Work out the finished part from the listing and answer in its coordinate system (mm). A direction names the side the tool comes from. Round coordinates to 2 decimals unless told otherwise and drop trailing zeros.
```python
from build123d import *

# Parameters (mm, degrees)
SKETCH2_W               = 316.892468242
SKETCH2_H               = 286.660554426
CUT_EXTRUDE1_DEPTH      = 1.27
CUT_EXTRUDE1_DEPTH_BACK = 77.2
SKETCH3_R               = 3.175
CUT_EXTRUDE2_DEPTH      = 19.05
CIRPATTERN1_COUNT       = 8


with BuildPart() as part:
    # Sketch1 → Revolve1 (revolve)
    with BuildSketch(Plane(origin=(0, 0, 0), x_dir=(0, 0, -1), z_dir=(1, 0, 0))):
        with BuildLine():
            ThreePointArc((-50.167050753, 76.2), (-43.047460251, 74.691369941), (-37.013141195, 70.623013134))
            Line((-37.013141195, 70.623013134), (-2.24506403, 35.85493597))
            ThreePointArc((-2.24506403, 35.85493597), (0, 34.925), (2.24506403, 35.85493597))
            ThreePointArc((2.24506403, 35.85493597), (21.675043526, 50.270960023), (44.45, 58.434734291))
            Line((44.45, 58.434734291), (44.45, 76.2))
            Line((44.45, 76.2), (30.1625, 76.2))
            Line((30.1625, 76.2), (30.1625, 73.025))
            Line((30.1625, 73.025), (25.4, 73.025))
            Line((25.4, 73.025), (25.4, 76.2))
            Line((25.4, 76.2), (-25.4, 76.2))
            Line((-25.4, 76.2), (-25.4, 73.025))
            Line((-25.4, 73.025), (-30.1625, 73.025))
            Line((-30.1625, 73.025), (-30.1625, 76.2))
            Line((-30.1625, 76.2), (-50.167050753, 76.2))
        make_face()
    revolve(axis=Axis((0, 0, 0), (0, 0, 1)))

    # Sketch2 → Cut-Extrude1 (cut, two sides)
    with BuildSketch(Plane(origin=(0, 0, 0), x_dir=(1, 0, 0), z_dir=(0, 1, 0))) as cut_extrude1_sk:
        Rectangle(SKETCH2_W, SKETCH2_H)
    extrude(amount=CUT_EXTRUDE1_DEPTH, mode=Mode.SUBTRACT)
    extrude(cut_extrude1_sk.sketch, amount=-CUT_EXTRUDE1_DEPTH_BACK, mode=Mode.SUBTRACT)

    # Sketch3 → Cut-Extrude2 (cut)
    with BuildSketch(Plane(origin=(29.160477546, 70.399620377, 0), x_dir=(0, 0, -1), z_dir=(0.382683432, 0.923879533, 0))):
        Circle(SKETCH3_R)
    cut_extrude2 = extrude(amount=-CUT_EXTRUDE2_DEPTH, mode=Mode.SUBTRACT)

    # CirPattern1: Cut-Extrude2 ×8 about axis
    cirpattern1_axis = Axis((0, 0, 0), (0, 0, 1))
    for i in range(1, CIRPATTERN1_COUNT):
        add(cut_extrude2.rotate(cirpattern1_axis, i * 360 / CIRPATTERN1_COUNT), mode=Mode.SUBTRACT)


solid = part.part
```
1. Given pin 1 (3 mm diameter, centred on y = 59, z = -35, fed in from -X); pin 2 (10 mm diameter, centred on x = -29, y = 32.5, fed in from -Z); pin 3 (4 mm diameter, centred on x = 31.5, y = 48.5, fed in from +Z), each flat-ended and moving along its own axis, determine where each tip first touches the part or whether it passes through.
Answer key:
pin 1: stops at x = -50
pin 2: stops at z = -18.63
pin 3: stops at z = 26.22
2. Which of the six approach directions +Z, -Z, +X, -X, +Y, -Y give full straight-line access (tool end or side, diameter ignored) to faces 4 (the face through (52.783, 21.911, 0.044)), 5 (the face through (0, 75, 25.4)), 6 (the face through (1.66, 76.18, 40.3))?
Answer key:
face 4: none
face 5: +Y
face 6: +Z, -Z, +Y
3. Determine the mould class of faces 1 (the face through (60, 1.27, -8)), 2 (the face through (-21.911, 52.783, 0.044)), 3 (the face through (1.588, 73.008, 27.815)) for opening direction X: +X half, -X half, draft (parallel to the pull), parting line (faces both ways), or undercut.
Answer key:
face 1: draft
face 2: undercut
face 3: parting line
4. Consider probe 1 along Z at (x, y) = (57, 46); probe 2 along Z at (x, y) = (-57, 23); probe 3 along Z at (x, y) = (60.5, 42). Determine where each line is inside the solid, lowest interval first.
Answer key:
probe 1: z = -44.45 to -30.16, -25.4 to 25.4, 30.16 to 40.29
probe 2: z = -44.45 to -3.12, 3.12 to 27.86
probe 3: z = -44.45 to -30.16, -25.4 to 25.4, 30.16 to 40.96
